Model file for the job. Use its own axes, mm. A direction names the side the tool comes from. Give positions to 0.01 mm unless a question says otherwise; leave off trailing zeros. Loops run counter-clockwise (first coordinate to the right, second up) from the corner with the lowest first, then second, coordinate; pieces in that order, holes last. Notation, with made-up numbers: M 39,72 L 83,72 A16 cw 83,102 Z; hole C 44,32 d10. An arc over 180 degrees is marked long. Answer in a Markdown table with one row per item.
```python
from build123d import *

# Parameters (mm, degrees)
SKETCH1_W           = 20
SKETCH1_H           = 15
BOSS_EXTRUDE1_DEPTH = 13
SKETCH2_R           = 2.5
BOSS_EXTRUDE2_DEPTH = 11.3
BOSS_EXTRUDE3_START = -7.5
SKETCH3_R           = 1.75
BOSS_EXTRUDE3_DEPTH = 10


with BuildPart() as part:
    # Sketch1 → Boss-Extrude1 (new body)
    with BuildSketch(Plane(origin=(0, 0, 0), x_dir=(0, 1, 0), z_dir=(0, 0, 1))):
        with Locations((-10, 7.5)):
            Rectangle(SKETCH1_W, SKETCH1_H)
    extrude(amount=BOSS_EXTRUDE1_DEPTH)

    # Sketch2 → Boss-Extrude2 (add)
    with BuildSketch(Plane.XZ.offset(20)):
        with Locations((-7.5, 6.5)):
            Circle(SKETCH2_R)
    extrude(amount=BOSS_EXTRUDE2_DEPTH)

    # Sketch3 → Boss-Extrude3 (add)
    with BuildSketch(Plane.YZ.offset(BOSS_EXTRUDE3_START)):
        with Locations((-29.55, 6.5)):
            Circle(SKETCH3_R)
        with Locations((-24.55, 6.5)):
            Circle(SKETCH3_R)
    extrude(amount=-BOSS_EXTRUDE3_DEPTH)


solid = part.part
```
(1) Wall check: L1, parallel to Y at x = -12.25, z = 6.25; L2, parallel to Y at x = -2, z = 5.25; L3, parallel to X at y = -15, z = 10.5. Give the ranges that are in metal, low to high.
Established:
| item | result |
|---|---|
| L1 | y = -31.28 to -27.82, -26.28 to -22.82, -20 to 0 |
| L2 | y = -20 to 0 |
| L3 | x = -15 to 0 |
(2) Mould opens along Y. For faces 1 (the flat face through (-7, 0, 6)), 2 (the flat face through (-7.4, -20, 3.5)), 3 (the flat face through (0, -10, 6)), 4 (the flat face through (-8, -31.3, 7)) say: pulls with the +Y half, pulls with the -Y half, needs draft (parallel to the pull), parting line crosses it, or undercut.
Established:
| item | result |
|---|---|
| face 1 | pulls with the +Y half |
| face 2 | undercut |
| face 3 | needs draft |
| face 4 | pulls with the -Y half |
(3) Saw through at B-B, the plane z = 5.75. Give the cut face in (x, y), and give its area (3 significant figures).
Established:
| item | result |
|---|---|
| outline | M -17.5,-31.13 L -9.88,-31.13 L -9.88,-31.3 L -5.12,-31.3 L -5.12,-20 L 0,-20 L 0,0 L -15,0 L -15,-20 L -9.88,-20 L -9.88,-22.97 L -17.5,-22.97 L -17.5,-26.13 L -9.88,-26.13 L -9.88,-27.97 L -17.5,-27.97 Z |
| area | 402 mm2 |
(4) Which spindle directions (+Z, -Z, +X, -X, +Y, -Y) get a long thin tool onto all of the face, cutting with end or side? Do faces 5 (the cylindrical face through (-5.115, -25.571, 7.251)), 6 (the flat face through (-17.5, -30, 7)), 7 (the flat face through (-8, -10, 13)), 8 (the cylindrical face through (-13.335, -22.933, 5.83)), 9 (the flat face through (-15, -10, 6)). Say none if no direction does.
Established:
| item | result |
|---|---|
| face 5 | none |
| face 6 | +Z, -Z, -X, +Y, -Y |
| face 7 | +Z, +X, -X, +Y, -Y |
| face 8 | -X |
| face 9 | +Z, -Z, -X, +Y |
(5) Saw through at D-D, the plane y = -29.55. Give the cut face in (x, z).
Established:
| item | result |
|---|---|
| outline | M -17.5,4.75 L -9.29,4.75 A2.5 ccw long -9.29,8.25 L -17.5,8.25 Z |
(6) Flat gauge pin, fed straight in: P1, Ø6.5, axis at y = -7.5, z = 4.5, coming from the -X side. Where does the tip first touch, or does it go through?
Established:
| item | result |
|---|---|
| P1 | stops at x = -15 |
(7) Saw through at A-A, the plane x = -13.25. Give the cut face in (y, z), and give its area (3 significant figures).
Established:
| item | result |
|---|---|
| outline | C -29.55,6.5 d3.5; C -24.55,6.5 d3.5; M -20,0 L 0,0 L 0,13 L -20,13 Z |
| area | 279 mm2 |
(8) Saw through at C-C, the plane x = -7.5. Give the cut face in (y, z).
Established:
| item | result |
|---|---|
| outline | M -31.3,4 L -20,4 L -20,0 L 0,0 L 0,13 L -20,13 L -20,9 L -31.3,9 Z |
